Check sheet for the modelled part. Datum: model origin and axes. Units: mm. A direction names the side the tool comes from. Round coordinates to 2 decimals unless told otherwise and drop trailing zeros. Order: outer loops, then holes, each group sorted by start corner. A loop starts at its lowest first (then second) coordinate and runs counter-clockwise, first axis right, second up.
Q1. Cross-section at B-B on x = 14. Record the cut outline in (y, z).
Q2. Depth check by flat-ended pin: P1, Ø0.7, axis at x = 37.5, y = 0.5, coming from the -Z side; P2, Ø0.6, axis at x = -45.5, z = -2, coming from the +Y side; P3, Ø2.5, axis at y = 7, z = -53.74, coming from the -X side. Enter the tip coordinate at first touch or a pass-through.
Q3. Set-up check for faces 1 (the flat face through (-45.89, 10.55, 4.98)), 2 (the flat face through (30.5, 13, -32)), 3 (the flat face through (45.89, 10.55, 4.98)): record each of +Z, -Z, +X, -X, +Y, -Y from which the full face is reachable in a straight line by a thin tool's end or side.
Q4. Cross-section at A-A on z = -31.5. Record the cut outline in (x, y), then the cut area to 3 significant figures.
Q5. Scan lines: probe 1 along X at (y, z) = (14, 0); probe 2 along Z at (x, y) = (20, 0.5); probe 3 along X at (y, z) = (0.5, -5). Record each from-to range of solid material in increasing order.
Q6. Mould release check, pull along Y, two halves, no side actions. Record for faces 4 (the conical face through (-41.1, 21.06, 9.51)), 5 (the cylindrical face through (36.437, 7.05, -54.867)), 6 (the flat face through (-45.914, 1.592, 0.049)): +Y half, -Y half, draft (parallel to the pull), parting line (faces both ways), or undercut.
from build123d import *

# Parameters (mm, degrees)
BOSS_EXTRUDE6_DEPTH            = 42.5
FILLET3_R                      = 4
BOSS_EXTRUDE7_DEPTH            = 19.200000225
SKETCH16_W                     = 12
SKETCH16_H                     = 56.251708931
BOSS_EXTRUDE8_DEPTH            = 21.200000225
MIRROR10_START                 = -2.25e-07
MIRROR10_DEPTH                 = 21.200000225
MIRROR10_START_2               = 19.2
MIRROR10_2_DEPTH               = 2
SKETCH17_R                     = 1.132230372
CUT_EXTRUDE3_DEPTH             = 109.502203117
CHAMFER1_SIZE                  = 0.5
SKETCH18_R                     = 5.5
CUT_EXTRUDE4_DEPTH             = 1.5
MIRROR12_COPY_1_SKETCH_R       = 5.5
MIRROR12_COPY_1_DEPTH          = 1.5
CUT_EXTRUDE7_REACH             = 100.98
CUT_EXTRUDE7_DIRECTION_2_REACH = 100.98
FILLET4_R                      = 4
SKETCH41_W                     = 5
SKETCH41_H                     = 0.8
BOSS_EXTRUDE20_DEPTH           = 0.6
BOSS_EXTRUDE21_DEPTH           = 3.5
BOSS_EXTRUDE23_DEPTH           = 2
FILLET5_R                      = 0.3
FILLET6_R                      = 0.1


# Read off the part's stored shape, not the designer's step: Mirror10
with BuildPart() as part:
    # Sketch14 → Boss-Extrude6 (new body)
    with BuildSketch(Plane(origin=(0, 0, 0), x_dir=(0, 0, -1), z_dir=(1, 0, 0))):
        Polygon((-7.766164208, -2.25e-07), (-10.966164208, -2.25e-07), (-10.966164208, 21.2), (10.966164208, 21.2), (10.966164208, -2.25e-07), (7.766164208, -2.25e-07), (7.766164208, 19.2), (-7.766164208, 19.2), align=None)
    extrude(amount=BOSS_EXTRUDE6_DEPTH)

    # Fillet3
    fillet3_edges = [part.edges().sort_by_distance(p)[0] for p in [
        (42.5, 10.599999888, 10.966164208),
    ]]
    fillet(fillet3_edges, radius=FILLET3_R)

    # Sketch15 → Boss-Extrude7 (add)
    with BuildSketch(Plane.XZ.offset(-19.2)):
        with BuildLine():
            Line((42.5, 6.966164208), (42.5, -7.766164208))
            Line((42.5, -7.766164208), (40, -7.766164208))
            Line((40, -7.766164208), (40, 6.966164208))
            ThreePointArc((40, 6.966164208), (39.99240423, 7.116927651), (39.969693846, 7.266164208))
            ThreePointArc((39.969693846, 7.266164208), (39.448683298, 8.128059212), (38.5, 8.466164208))
            Line((38.5, 8.466164208), (38.5, 10.966164208))
            ThreePointArc((38.5, 10.966164208), (41.029822128, 10.064550885), (42.419183588, 7.766164208))
            ThreePointArc((42.419183588, 7.766164208), (42.479744612, 7.368200056), (42.5, 6.966164208))
        make_face()
    extrude(amount=BOSS_EXTRUDE7_DEPTH)

    # Sketch16 → Boss-Extrude8 (add)
    with BuildSketch(Plane(origin=(0, 21.2, 0), x_dir=(1, 0, 0), z_dir=(0, 1, 0))):
        with Locations((36.5, 35.892018674)):
            Rectangle(SKETCH16_W, SKETCH16_H)
    extrude(amount=-BOSS_EXTRUDE8_DEPTH)

    # Mirror10 outline → Mirror10 (add)
    with BuildSketch(Plane(origin=(0, 0, 0), x_dir=(1, 0, 0), z_dir=(0, 1, 0)).offset(MIRROR10_START)):
        with BuildLine():
            Line((0, -7.766164208), (-39.768857754, -7.766164208))
            ThreePointArc((-39.768857754, -7.766164208), (-39.941056319, -7.382525451), (-40, -6.966164208))
            Line((-40, -6.966164208), (-40, 7.766164208))
            Line((-40, 7.766164208), (0, 7.766164208))
            Line((0, 7.766164208), (0, 10.966164208))
            Line((0, 10.966164208), (-30.5, 10.966164208))
            Line((-30.5, 10.966164208), (-30.5, 64.017873139))
            Line((-30.5, 64.017873139), (-42.5, 64.017873139))
            Line((-42.5, 64.017873139), (-42.5, -6.966164208))
            ThreePointArc((-42.5, -6.966164208), (-41.328427125, -9.794591333), (-38.5, -10.966164208))
            Line((-38.5, -10.966164208), (0, -10.966164208))
            Line((0, -10.966164208), (0, -7.766164208))
        make_face()
    extrude(amount=MIRROR10_DEPTH)

    # Mirror10 2 outline → Mirror10 2 (add)
    with BuildSketch(Plane(origin=(0, 0, 0), x_dir=(1, 0, 0), z_dir=(0, 1, 0)).offset(MIRROR10_START_2)):
        with BuildLine():
            ThreePointArc((-40, -6.966164208), (-39.941056319, -7.382525451), (-39.768857754, -7.766164208))
            Line((-39.768857754, -7.766164208), (0, -7.766164208))
            Line((0, -7.766164208), (0, 7.766164208))
            Line((0, 7.766164208), (-40, 7.766164208))
            Line((-40, 7.766164208), (-40, -6.966164208))
        make_face()
    extrude(amount=MIRROR10_2_DEPTH)

    # Sketch17 → Cut-Extrude3 (cut, through all)
    with BuildSketch(Plane.ZY.offset(42.5)):
        with Locations((-53.736263186, 6.999999775)):
            Circle(SKETCH17_R)
        with BuildLine():
            Line((-9.466164208, 21.2), (-54.264633471, 8.928943746))
            ThreePointArc((-54.264633471, 8.928943746), (-55.665207156, 6.47162949), (-53.207892901, 5.071055805))
            Line((-53.207892901, 5.071055805), (-16.022904778, 15.256651174))
            ThreePointArc((-16.022904778, 15.256651174), (-12.539949284, 14.578933218), (-10.966164208, 11.398763232))
            Line((-10.966164208, 11.398763232), (-10.966164208, -2.25e-07))
            Line((-10.966164208, -2.25e-07), (-58.949878023, -2.25e-07))
            Line((-58.949878023, -2.25e-07), (-64.017873139, -2.25e-07))
            Line((-64.017873139, -2.25e-07), (-64.017873139, 6.372862294))
            Line((-64.017873139, 6.372862294), (-64.017873139, 21.2))
            Line((-64.017873139, 21.2), (-9.466164208, 21.2))
        make_face()
    extrude(amount=-CUT_EXTRUDE3_DEPTH, mode=Mode.SUBTRACT)

    # Chamfer1
    chamfer1_edges = [part.edges().sort_by_distance(p)[0] for p in [
        (-42.5, 21.2, -1.25),
        (42.5, 21.2, -1.25),
        (19.25, 21.2, 10.966164208),
        (41.328427125, 21.2, 9.794591333),
        (-41.328427125, 21.2, 9.794591333),
    ]]
    chamfer(chamfer1_edges, length=CHAMFER1_SIZE)

    # Sketch18 → Cut-Extrude4 (cut)
    with BuildSketch(Plane.ZY.offset(42.5)):
        with Locations((-53.736263186, 6.999999775)):
            Circle(SKETCH18_R)
    cut_extrude4 = extrude(amount=-CUT_EXTRUDE4_DEPTH, mode=Mode.SUBTRACT)

    # Mirror11: Cut-Extrude4 across plane
    add(cut_extrude4.mirror(Plane.ZY.offset(36.5)), mode=Mode.SUBTRACT)

    # Mirror12: Cut-Extrude4 across plane
    add(cut_extrude4.mirror(Plane(origin=(0, 0, 0), x_dir=(0, 0, 1), z_dir=(1, 0, 0))), mode=Mode.SUBTRACT)

    # Mirror12 copy 1 sketch → Mirror12 copy 1 (cut)
    with BuildSketch(Plane.ZY.offset(-30.5)):
        with Locations((-53.736263186, 6.999999775)):
            Circle(MIRROR12_COPY_1_SKETCH_R)
    extrude(amount=-MIRROR12_COPY_1_DEPTH, mode=Mode.SUBTRACT)

    # Cut-Extrude7: up to this face of the body (flat: up to its plane)
    cut_extrude7_end = Plane(part.part.faces().sort_by_distance((-40, 9.599999887, -0.4))[0])
    # Sketch23 → Cut-Extrude7 (cut, up to the picked face)
    with BuildSketch(Plane.ZY.offset(36.5), mode=Mode.PRIVATE) as cut_extrude7_sk1:
        with BuildLine():
            Line((-16.287089921, 16.221123159), (-45.347315212, 8.261037353))
            ThreePointArc((-45.347315212, 8.261037353), (-45.878172566, 7.903119099), (-46.083130069, 7.296565368))
            Line((-46.083130069, 7.296565368), (-46.083130069, 7.022648503))
            Line((-46.083130069, 7.022648503), (-47.68348017, 6.584285621))
            Line((-47.68348017, 6.584285621), (-47.68348017, 7.406036215))
            ThreePointArc((-47.68348017, 7.406036215), (-47.068607659, 9.225697409), (-45.476035597, 10.299452171))
            Line((-45.476035597, 10.299452171), (-11.027350425, 19.735528015))
            Line((-11.027350425, 19.735528015), (-7.766164208, 19.2))
            Line((-7.766164208, 19.2), (-7.766164208, 13.2))
            Line((-7.766164208, 13.2), (-10.301880115, 13.2))
            ThreePointArc((-10.301880115, 13.2), (-12.713097942, 15.862359585), (-16.287089921, 16.221123159))
        make_face()
    cut_extrude7_tool1 = split(extrude(cut_extrude7_sk1.sketch, amount=CUT_EXTRUDE7_REACH, mode=Mode.PRIVATE), bisect_by=cut_extrude7_end, keep=Keep.BOTH, mode=Mode.PRIVATE)
    add(cut_extrude7_tool1.solids().sort_by(Axis((-36.5, 14.283351, -24.707146), (-1, 0, 0)))[0], mode=Mode.SUBTRACT)

    # Cut-Extrude7 direction 2: up to this face of the body (flat: up to its plane)
    cut_extrude7_direction_2_end = Plane(part.part.faces().sort_by_distance((-32, 7.583720498, -51.605249006))[0])
    # Sketch23 → Cut-Extrude7 direction 2 (cut, up to the picked face)
    with BuildSketch(Plane.ZY.offset(36.5), mode=Mode.PRIVATE) as cut_extrude7_direction_2_sk1:
        with BuildLine():
            Line((-16.287089921, 16.221123159), (-45.347315212, 8.261037353))
            ThreePointArc((-45.347315212, 8.261037353), (-45.878172566, 7.903119099), (-46.083130069, 7.296565368))
            Line((-46.083130069, 7.296565368), (-46.083130069, 7.022648503))
            Line((-46.083130069, 7.022648503), (-47.68348017, 6.584285621))
            Line((-47.68348017, 6.584285621), (-47.68348017, 7.406036215))
            ThreePointArc((-47.68348017, 7.406036215), (-47.068607659, 9.225697409), (-45.476035597, 10.299452171))
            Line((-45.476035597, 10.299452171), (-11.027350425, 19.735528015))
            Line((-11.027350425, 19.735528015), (-7.766164208, 19.2))
            Line((-7.766164208, 19.2), (-7.766164208, 13.2))
            Line((-7.766164208, 13.2), (-10.301880115, 13.2))
            ThreePointArc((-10.301880115, 13.2), (-12.713097942, 15.862359585), (-16.287089921, 16.221123159))
        make_face()
    cut_extrude7_direction_2_tool1 = split(extrude(cut_extrude7_direction_2_sk1.sketch, amount=-CUT_EXTRUDE7_DIRECTION_2_REACH, mode=Mode.PRIVATE), bisect_by=cut_extrude7_direction_2_end, keep=Keep.BOTH, mode=Mode.PRIVATE)
    add(cut_extrude7_direction_2_tool1.solids().sort_by(Axis((-36.5, 14.283351, -24.707146), (1, 0, 0)))[0], mode=Mode.SUBTRACT)

    # Fillet4
    fillet4_edges = [part.edges().sort_by_distance(p)[0] for p in [
        (-30.5, 16.093943968, -10.966164208),
        (30.5, 16.093943967, -10.966164208),
    ]]
    fillet(fillet4_edges, radius=FILLET4_R)

    # Sketch41 → Boss-Extrude20 (add)
    with BuildSketch(Plane.XZ):
        Polygon((-40, -5.266164208), (-35, -6.966164208), (-35, -7.766164208), (-40, -7.766164208), align=None)
        Polygon((35, -6.966164208), (35, -7.766164208), (40, -7.766164208), (40, -5.266164208), align=None)
        with Locations((-37.5, 7.366164208)):
            Rectangle(SKETCH41_W, SKETCH41_H)
        with Locations((37.5, 7.366164208)):
            Rectangle(SKETCH41_W, SKETCH41_H)
    extrude(amount=-BOSS_EXTRUDE20_DEPTH)

    # Sketch42 → Boss-Extrude21 (add, symmetric)
    with BuildSketch(Plane.XY):
        Polygon((-44.9, 0.143703762), (-44.9, -4.017561374), (-43.1, -4.017561374), (-41.65, -1.517561374), (-42.8, -0.682037466), (-42.8, 7.995486209), (-42.5, 8.363098451), (-42.5, 13.2), (-44.3, 7.840797374), (-44.3, 4.199999775), (-44.9, 4.199999775), (-44.9, 2.999999775), (-46.9, 2.999999775), align=None)
    boss_extrude21 = extrude(amount=BOSS_EXTRUDE21_DEPTH, both=True)

    # Sketch44 → Boss-Extrude23 (add)
    with BuildSketch(Plane.ZY.offset(44.9)):
        with BuildLine():
            Line((-3.5, 2.999999775), (3.5, 2.999999775))
            Line((3.5, 2.999999775), (6.499239291, 18.315643504))
            ThreePointArc((6.499239291, 18.315643504), (6.080655383, 19.971079661), (4.536519218, 20.7))
            Line((4.536519218, 20.7), (-4.536519218, 20.7))
            ThreePointArc((-4.536519218, 20.7), (-6.080655383, 19.971079661), (-6.499239291, 18.315643504))
            Line((-6.499239291, 18.315643504), (-3.5, 2.999999775))
        make_face()
    boss_extrude23 = extrude(amount=BOSS_EXTRUDE23_DEPTH)

    # Mirror13: Boss-Extrude21, Boss-Extrude23 across plane
    add(boss_extrude21.mirror(Plane(origin=(0, 0, 0), x_dir=(0, 0, 1), z_dir=(1, 0, 0))))
    add(boss_extrude23.mirror(Plane(origin=(0, 0, 0), x_dir=(0, 0, 1), z_dir=(1, 0, 0))))

    # Fillet5
    fillet5_edges = [part.edges().sort_by_distance(p)[0] for p in [
        (-44.9, 4.199999775, 0),
        (-44.3, 4.199999775, 0),
    ]]
    fillet(fillet5_edges, radius=FILLET5_R - 0.0001)  # a hair under: the kernel refuses the full size

    # Fillet6
    fillet6_edges = [part.edges().sort_by_distance(p)[0] for p in [
        (-42.5, 8.363098451, 0),
    ]]
    fillet(fillet6_edges, radius=FILLET6_R)


solid = part.part
Results found:
1. outline: (0, -10.97) - (20.79, -10.97) - (21.2, -9.47) - (21.2, 10.47) - (20.7, 10.97) - (0, 10.97) - (0, 7.77) - (19.2, 7.77) - (19.2, -7.77) - (0, -7.77) - close
2. P1: stops at z = -10.97
2. P2: stops at y = 20.7
2. P3: stops at x = -41
3. face 1: +Z, -X, -Y
3. face 2: -Z, +Y, -Y
3. face 3: +Z, +X, -Y
4. outline: (-42.5, 11.02) - (-30.5, 11.02) - (-30.5, 15.16) - (-42.5, 15.16) - close; (30.5, 11.02) - (42.5, 11.02) - (42.5, 15.16) - (30.5, 15.16) - close; hole (-40, 12.05) - (-32, 12.05) - (-32, 14.13) - (-40, 14.13) - close
4. area: 82.9 mm2
5. probe 1: x = -46.9 to -44.9, -42.5 to -40, 40 to 42.5, 44.9 to 46.9
5. probe 2: z = -10.97 to -7.77, 7.77 to 10.97
5. probe 3: x = -42.5 to -40, 40 to 42.5
6. face 4: +Y half
6. face 5: undercut
6. face 6: -Y half
